Can you work these out from the model? Positions are in its coordinate system, mm. A direction names the side the tool comes from. Give positions to 0.01 mm unless a question says otherwise; leave off trailing zeros. Write each loop counter-clockwise with the first axis right and the second up, starting at its lowest first coordinate (ties: lowest second). Pieces come first, ordered by that corner, then holes.
```python
from build123d import *

# Parameters (mm, degrees)
SKETCH1_R               = 9
BOSS_EXTRUDE1_DEPTH     = 300
CUT_EXTRUDE1_DEPTH      = 301.269878609
CUT_EXTRUDE1_DEPTH_BACK = 301.269878609
SKETCH3_W               = 149.9
SKETCH3_H               = 5
BOSS_EXTRUDE2_DEPTH     = 300
CUT_EXTRUDE2_DEPTH      = 338.338109321
CUT_EXTRUDE2_DEPTH_BACK = 338.338109321


with BuildPart() as part:
    # Sketch1 → Boss-Extrude1 (new body)
    with BuildSketch(Plane(origin=(0, 0, 0), x_dir=(0, 0, -1), z_dir=(1, 0, 0))):
        Circle(SKETCH1_R)
    extrude(amount=BOSS_EXTRUDE1_DEPTH)

    # Sketch2 → Cut-Extrude1 (cut, two sides: drawn at the far end of the back side and taken through both)
    with BuildSketch(Plane(origin=(300, 0, 0), x_dir=(0, 0, -1), z_dir=(1, 0, 0)).offset(-CUT_EXTRUDE1_DEPTH_BACK)):
        with BuildLine():
            Line((-2.563201124, 3.2), (2.563201124, 3.2))
            ThreePointArc((2.563201124, 3.2), (0, -4.1), (-2.563201124, 3.2))
        make_face()
    extrude(amount=CUT_EXTRUDE1_DEPTH + CUT_EXTRUDE1_DEPTH_BACK, mode=Mode.SUBTRACT)

    # Sketch3 → Boss-Extrude2 (add)
    with BuildSketch(Plane(origin=(300, 0, 0), x_dir=(0, 0, -1), z_dir=(1, 0, 0))):
        with Locations((79.05, 0)):
            Rectangle(SKETCH3_W, SKETCH3_H)
    extrude(amount=-BOSS_EXTRUDE2_DEPTH)

    # Sketch4 → Cut-Extrude2 (cut, two sides: drawn at the far end of the back side and taken through both)
    with BuildSketch(Plane(origin=(300, 0, 0), x_dir=(0, 0, -1), z_dir=(1, 0, 0)).offset(-CUT_EXTRUDE2_DEPTH_BACK)):
        with BuildLine():
            Line((154, 2.5), (151.5, 2.5))
            ThreePointArc((151.5, 2.5), (153.267766953, 1.767766953), (154, 0))
            Line((154, 0), (154, 2.5))
        make_face()
        with BuildLine():
            Line((154, -2.5), (154, 0))
            ThreePointArc((154, 0), (153.267766953, -1.767766953), (151.5, -2.5))
            Line((151.5, -2.5), (154, -2.5))
        make_face()
    extrude(amount=CUT_EXTRUDE2_DEPTH + CUT_EXTRUDE2_DEPTH_BACK, mode=Mode.SUBTRACT)


solid = part.part
```
1) Suppose I cut it at C-C on y = 6. Write out the boundary of the cut face in (x, z).
Values follow:
outline: (0, -6.71) - (300, -6.71) - (300, 6.71) - (0, 6.71) - close
2) For pin 1 Ø1.5 at (x, z) = (127.5, -48) entering from -Y; pin 2 Ø4 at (x, y) = (66.5, -5) entering from -Z; pin 3 Ø6 at (x, z) = (203, -91.5) entering from +Y, each with a flat end and sliding along its axis, tell me the tip position at first contact or that it passes through.
Values follow:
pin 1: stops at y = -2.5
pin 2: stops at z = -8.49
pin 3: stops at y = 2.5
3) If we mould it in two halves opening along Z, with no side actions, what happens to faces 4 (the face through (148, 0, 9)), 5 (the face through (300, 0, -60)), 6 (the face through (147.9, -4.1, -0.1))? For each: +Z half, -Z half, draft (parallel to the pull), parting line (faces both ways), or undercut.
Values follow:
face 4: parting line
face 5: draft
face 6: undercut
4) Please list where these lines run through material, in increasing order: L1, parallel to Y at x = 138, z = 0; L2, parallel to Z at x = 234.5, y = -0.5; L3, parallel to Y at x = 170, z = -98.5.
Values follow:
L1: y = -9 to -4.1, 3.2 to 9
L2: z = -153.95 to -4.07, 4.07 to 8.99
L3: y = -2.5 to 2.5
5) Suppose I cut it at A-A on x = 105.5. Write out the boundary of the cut face in (y, z), plus the area to 3 significant figures.
Values follow:
outline: (-2.5, -151.5) arc R2.5 ccw to (2.5, -151.5) - (2.5, -8.65) arc R9 ccw (long way) to (-2.5, -8.65) - close; hole (3.2, -2.56) - (3.2, 2.56) arc R4.1 ccw (long way) to start
area: 928 mm2
6) Suppose I cut it at B-B on z = -84.5. Write out the boundary of the cut face in (x, y), plus the area to 3 significant figures.
Values follow:
outline: (0, -2.5) - (300, -2.5) - (300, 2.5) - (0, 2.5) - close
area: 1,500 mm2
7) For faces 1 (the face through (152, -2.5, -79)), 2 (the face through (152, 2.5, -79)), 3 (the face through (0, 0, -60)), which set-ups out of +Z, -Z, +X, -X, +Y, -Y let a thin tool reach every point of the face, with its end or its side?
Values follow:
face 1: -Z, +X, -X, -Y
face 2: -Z, +X, -X, +Y
face 3: +Z, -Z, -X, +Y, -Y
